Verification items for the finished model (mm, model axes). A direction names the side the tool comes from. Give positions to 0.01 mm unless a question says otherwise; leave off trailing zeros. Write each loop counter-clockwise with the first axis right and the second up, starting at its lowest first coordinate (ties: lowest second). Pieces come first, ordered by that corner, then holes. Notation, with made-up numbers: (-23, 62.5) -> (12, 62.5) arc R24 cw to (12, 87.5) -> close; hole circle Ø9 at (-12.75, 32.5). An arc over 180 degrees is marked (long way). Write item = value, one per line.
from build123d import *

# Parameters (mm, degrees)
F0_W     = 17
F0_H     = 10
F1_DEPTH = 17
F2_W     = 5
F2_H     = 10
F2_R     = 3.5
F3_DEPTH = 12.5
F4_R     = 1.5
F5_DEPTH = 20


with BuildPart() as f1:
    # F0 (on Front) → F1 (new body)
    with BuildSketch(Plane.XZ):
        Rectangle(F0_W, F0_H)
        Polygon((8.5, -5), (-8.5, -5), (-12.5, -5), (-12.5, -29), (-8.5, -29), (-8.5, -11), (8.5, -11), (8.5, -29), (12.5, -29), (12.5, -5), align=None)
    extrude(amount=F1_DEPTH)

    # F2 (on Right) → F3 (cut, symmetric)
    with BuildSketch(Plane.YZ):
        with Locations((-2.5, 0.153744)):
            Rectangle(F2_W, F2_H)
        with Locations((-8.5, -19)):
            Circle(F2_R)
    extrude(amount=F3_DEPTH, both=True, mode=Mode.SUBTRACT)

    # F4 (on Top) → F5 (cut, symmetric)
    with BuildSketch(Plane.XY):
        with Locations((0, -11)):
            Circle(F4_R)
    extrude(amount=F5_DEPTH, both=True, mode=Mode.SUBTRACT)


solid = f1.part
Item 1: Sectioned sample at D-D on z = -19. Record the cut outline in (x, y), then the cut area to 3 significant figures.
Response values:
outline = (-12.5, -17) -> (-8.5, -17) -> (-8.5, -12) -> (-12.5, -12) -> close; (-12.5, -5) -> (-8.5, -5) -> (-8.5, 0) -> (-12.5, 0) -> close; (8.5, -17) -> (12.5, -17) -> (12.5, -12) -> (8.5, -12) -> close; (8.5, -5) -> (12.5, -5) -> (12.5, 0) -> (8.5, 0) -> close
area = 80.0 mm^2
Item 2: Sectioned sample at C-C on y = -8.5. Record the cut outline in (x, z).
Response values:
outline = (-12.5, -29) -> (-8.5, -29) -> (-8.5, -22.5) -> (-12.5, -22.5) -> close; (-12.5, -15.5) -> (-8.5, -15.5) -> (-8.5, -11) -> (8.5, -11) -> (8.5, -15.5) -> (12.5, -15.5) -> (12.5, -5) -> (8.5, -5) -> (8.5, 5) -> (-8.5, 5) -> (-8.5, -5) -> (-12.5, -5) -> close; (8.5, -29) -> (12.5, -29) -> (12.5, -22.5) -> (8.5, -22.5) -> close
Item 3: Sectioned sample at B-B on x = 0. Record the cut outline in (y, z).
Response values:
outline = (-17, -11) -> (-12.5, -11) -> (-12.5, 5) -> (-17, 5) -> close; (-9.5, -11) -> (0, -11) -> (0, -4.85) -> (-5, -4.85) -> (-5, 5) -> (-9.5, 5) -> close
Item 4: Set-up check for faces 1 (the flat face through (8.5, -6, -22)), 2 (the flat face through (-8.5, -10, 0)), 3 (the cylindrical face through (-0.325, -12.464, -2.888)), 4 (the flat face through (8.5, -10, 0)), 5 (the flat face through (0, -3, -4.846)): record each of +Z, -Z, +X, -X, +Y, -Y from which the full face is reachable in a straight line by a thin tool's end or side.
Response values:
face_1 = -Z, +Y, -Y
face_2 = +Z, -X, +Y, -Y
face_3 = +Z, -Z
face_4 = +Z, +X, +Y, -Y
face_5 = +Z, +X, -X, +Y
Item 5: Mould release check, pull along Z, two halves, no side actions. Record for faces 6 (the flat face through (0, -17, -8)), 7 (the cylindrical face through (10.528, -11.08, -16.635)), 8 (the flat face through (-10, -8, -5)), 9 (the flat face through (10, -8, -29)): +Z half, -Z half, draft (parallel to the pull), parting line (faces both ways), or undercut.
Response values:
face_6 = draft
face_7 = undercut
face_8 = +Z half
face_9 = -Z half
Item 6: Material ranges on line 1 (Y direction, x = 0, z = 0); line 2 (X direction, y = -12.5, z = -26); line 3 (Z direction, x = 10.45, y = -8.5), recorded low to high.
Response values:
line_1 = -17 to -12.5, -9.5 to -5
line_2 = -12.5 to -8.5, 8.5 to 12.5
line_3 = -29 to -22.5, -15.5 to -5
Item 7: Go/stop test with flat-tipped pins: P1, Ø5, axis at x = -1, y = -5, coming from the -Z side; P2, Ø2, axis at x = 3.5, y = -2.5, coming from the +Z side; P3, Ø3, axis at y = -4.5, z = 1.5, coming from the +X side; P4, Ø4, axis at y = -8.5, z = -19, coming from the +X side. Record where each tip stops, or that it passes through.
Response values:
P1 = -11
P2 = -4.85
P3 = 8.5
P4 = through
Item 8: Sectioned sample at A-A on z = -23.5. Record the cut outline in (x, y), then the cut area to 3 significant figures.
Response values:
outline = (-12.5, -17) -> (-8.5, -17) -> (-8.5, 0) -> (-12.5, 0) -> close; (8.5, -17) -> (12.5, -17) -> (12.5, 0) -> (8.5, 0) -> close
area = 136 mm^2
